Source: CAD feature listing. Evaluate the final solid. Frame: model axes, mm. A direction names the side the tool comes from. Round coordinates to 2 decimals unless told otherwise and drop trailing zeros. Write each loop counter-clockwise with the first axis right and the second up, starting at its lowest first coordinate (ties: lowest second). Pieces come first, ordered by that corner, then holes.
from build123d import *

# Parameters (mm, degrees)
ESQUISSE1_W             = 100
ESQUISSE1_H             = 65
BOSS_EXTRU_1_DEPTH      = 5
ESQUISSE2_W             = 15
ESQUISSE2_H             = 5.01
ESQUISSE2_W_2           = 15.01
ESQUISSE2_W_3           = 14.51
ESQUISSE2_W_4           = 5
ESQUISSE2_H_2           = 17.5
ENL_V_MAT_EXTRU_1_DEPTH = 5
ESQUISSE3_R             = 7.505
ENL_V_MAT_EXTRU_2_DEPTH = 10


with BuildPart() as part:
    # Esquisse1 → Boss.-Extru.1 (new body)
    with BuildSketch(Plane.XY):
        Rectangle(ESQUISSE1_W, ESQUISSE1_H)
    extrude(amount=BOSS_EXTRU_1_DEPTH)

    # Esquisse2 → Enlèv. mat.-Extru.1 (cut)
    with BuildSketch(Plane.XY.offset(5)):
        with Locations((-42.5, 29.995)):
            Rectangle(ESQUISSE2_W, ESQUISSE2_H)
        with Locations((-14.005, 29.995)):
            Rectangle(ESQUISSE2_W_2, ESQUISSE2_H)
        with Locations((14.495, 29.995)):
            Rectangle(ESQUISSE2_W_2, ESQUISSE2_H)
        with Locations((42.745, 29.995)):
            Rectangle(ESQUISSE2_W_3, ESQUISSE2_H)
        with Locations((-47.5, 0.25)):
            Rectangle(ESQUISSE2_W_4, ESQUISSE2_H_2)
        with Locations((47.5, 0.25)):
            Rectangle(ESQUISSE2_W_4, ESQUISSE2_H_2)
        with Locations((42.745, -29.995)):
            Rectangle(ESQUISSE2_W_3, ESQUISSE2_H)
        with Locations((14.495, -29.995)):
            Rectangle(ESQUISSE2_W_2, ESQUISSE2_H)
        with Locations((-14.005, -29.995)):
            Rectangle(ESQUISSE2_W_2, ESQUISSE2_H)
        with Locations((-42.5, -29.995)):
            Rectangle(ESQUISSE2_W, ESQUISSE2_H)
    extrude(amount=-ENL_V_MAT_EXTRU_1_DEPTH, mode=Mode.SUBTRACT)

    # Esquisse3 → Enlèv. mat.-Extru.2 (cut)
    with BuildSketch(Plane.XY.offset(5)):
        with Locations((-12, -13)):
            Circle(ESQUISSE3_R)
        with BuildLine():
            Line((6.973645564, 21.746445448), (9.973645564, 23.199570448))
            ThreePointArc((9.973645564, 23.199570448), (40.699570448, 12.526354436), (30.026354436, -18.199570448))
            Line((30.026354436, -18.199570448), (27.026354436, -19.652695448))
            ThreePointArc((27.026354436, -19.652695448), (-3.699570448, -8.979479436), (6.973645564, 21.746445448))
        make_face()
    extrude(amount=-ENL_V_MAT_EXTRU_2_DEPTH, mode=Mode.SUBTRACT)


solid = part.part
1) Material intervals for line 1 (X direction, y = 29, z = 3.45); line 2 (Y direction, x = -12, z = 2.2) (3 decimals); line 3 (X direction, y = -10.5, z = 2.4), sorted ascending.
Taken from the geometry:
line 1: x = -35 to -21.51, -6.5 to 6.99, 22 to 35.49
line 2: y = -27.49 to -20.505, -5.495 to 27.49
line 3: x = -50 to -19.08, -4.92 to -2.89, 38.97 to 50
2) Pull-direction query (Y, two-part tool) for faces 5 (the face through (-14, 27.49, 3)), 6 (the face through (-48, 9, 3)), 7 (the face through (14, -27.49, 3)), 8 (the face through (-21.51, -30, 3)); classes: released by +Y, released by -Y, zero draft, split by the parting line, or undercut.
Taken from the geometry:
face 5: released by +Y
face 6: undercut
face 7: released by -Y
face 8: zero draft
3) Section query A-A on x = -12. Return the cut outline in (y, z) (3 decimals), then the cut area to 3 significant figures.
Taken from the geometry:
outline: (-27.49, 0) - (-20.505, 0) - (-20.505, 5) - (-27.49, 5) - close; (-5.495, 0) - (27.49, 0) - (27.49, 5) - (-5.495, 5) - close
area: 200 mm2
4) Section query B-B on y = 19. Return the cut outline in (x, z), then the cut area to 3 significant figures.
Taken from the geometry:
outline: (-50, 0) - (2.62, 0) - (2.62, 5) - (-50, 5) - close; (36.02, 0) - (50, 0) - (50, 5) - (36.02, 5) - close
area: 333 mm2
5) Contact query for flat-ended pins moving along their axis: P1, Ø3, axis at y = 5.5, z = 2.5, coming from the -X side; P2, Ø2.5, axis at x = 15.5, z = 3, coming from the -Y side; P3, Ø2.5, axis at y = -29, z = 2.5, coming from the +X side. Output: stop coordinate, or through.
Taken from the geometry:
P1: stops at x = -45
P2: stops at y = -27.49
P3: stops at x = 35.49
6) Section query C-C on z = 1.1. State how many separate pieces and enclosed holes the cut face has, then the cut area to 3 significant figures.
Taken from the geometry:
separate pieces: 1
enclosed holes: 2
area: 3,740 mm2
7) Section query D-D on x = -40.5. Return the cut outline in (y, z).
Taken from the geometry:
outline: (-27.49, 0) - (27.49, 0) - (27.49, 5) - (-27.49, 5) - close
8) Reachability of faces 1 (the face through (8.45, 22.46, 2.54)), 2 (the face through (43, -27.49, 3)), 3 (the face through (22, 30, 3)), 4 (the face through (47, -8.5, 3)) from +Z, -Z, +X, -X, +Y, -Y: full face, straight path, thin tool, end or side. Return the list, or none.
Taken from the geometry:
face 1: +Z, -Z
face 2: +Z, -Z, +X, -Y
face 3: +Z, -Z, +Y
face 4: +Z, -Z, +X
